```python
from build123d import *

# Parameters (mm, degrees)
SKETCH3_W            = 100
SKETCH3_H            = 120
BOSS_EXTRUDE3_DEPTH  = 4
M4_CLEARANCE_HOLE1_D = 4.5
SKETCH5_R            = 11.8
CUT_EXTRUDE3_DEPTH   = 79.204859184
FILLET1_R            = 15
SKETCH23_W           = 9
SKETCH23_H           = 10
BOSS_EXTRUDE5_DEPTH  = 10
SKETCH26_W           = 40
SKETCH26_H           = 2
BOSS_EXTRUDE6_DEPTH  = 3
SKETCH27_R           = 2.3
CUT_EXTRUDE4_DEPTH   = 6.6
CUT_EXTRUDE5_START   = -6.6
SKETCH28_R           = 2.3
CUT_EXTRUDE5_DEPTH   = 6.6
FILLET2_R            = 2
FILLET3_R            = 2
FILLET4_R            = 2
FILLET5_R            = 2
FILLET6_R            = 2
FILLET7_R            = 2


with BuildPart() as part:
    # Sketch3 → Boss-Extrude3 (new body)
    with BuildSketch(Plane(origin=(0, 0, 0), x_dir=(1, 0, 0), z_dir=(0, 1, 0))):
        Rectangle(SKETCH3_W, SKETCH3_H)
    extrude(amount=BOSS_EXTRUDE3_DEPTH)

    # M4 Clearance Hole1 (through all)
    with Locations(Plane(origin=(0, 4, 0), x_dir=(1, 0, 0), z_dir=(0, 1, 0))):
        with Locations((-8.35, -18.35), (-39.35, -18.35), (-39.35, -49.35), (-8.35, -49.35), (8.35, -18.35), (39.35, -18.35), (39.35, -49.35), (8.35, -49.35)):
            Hole(M4_CLEARANCE_HOLE1_D / 2)

    # Sketch5 → Cut-Extrude3 (cut, through all)
    with BuildSketch(Plane(origin=(0, 4, 0), x_dir=(1, 0, 0), z_dir=(0, 1, 0))):
        with Locations(Location((-23.85, -33.85, 0), (0, 0, 270))):
            Circle(SKETCH5_R)
        with Locations(Location((23.85, -33.85, 0), (0, 0, 270))):
            Circle(SKETCH5_R)
    extrude(amount=-CUT_EXTRUDE3_DEPTH, mode=Mode.SUBTRACT)

    # Fillet1
    fillet1_edges = [part.edges().sort_by_distance(p)[0] for p in [
        (50, 2, 60),
        (-50, 2, 60),
        (-50, 2, -60),
        (50, 2, -60),
    ]]
    fillet(fillet1_edges, radius=FILLET1_R)

    # Sketch23 → Boss-Extrude5 (add)
    with BuildSketch(Plane.XZ):
        with Locations((-42.5, -40)):
            Rectangle(SKETCH23_W, SKETCH23_H)
        with Locations((42.5, -40)):
            Rectangle(SKETCH23_W, SKETCH23_H)
    extrude(amount=BOSS_EXTRUDE5_DEPTH)

    # Sketch26 → Boss-Extrude6 (add)
    with BuildSketch(Plane.XZ):
        with Locations((0, 58)):
            Rectangle(SKETCH26_W, SKETCH26_H)
    extrude(amount=BOSS_EXTRUDE6_DEPTH)

    # Sketch27 → Cut-Extrude4 (cut)
    with BuildSketch(Plane.ZY.offset(47)):
        with Locations((-40, -5)):
            Circle(SKETCH27_R)
    extrude(amount=-CUT_EXTRUDE4_DEPTH, mode=Mode.SUBTRACT)

    # Sketch28 → Cut-Extrude5 (cut)
    with BuildSketch(Plane(origin=(47, 0, 0), x_dir=(0, 0, -1), z_dir=(1, 0, 0)).offset(CUT_EXTRUDE5_START)):
        with Locations(Location((40, -5, 0), (0, 0, 180))):
            Circle(SKETCH28_R)
    extrude(amount=CUT_EXTRUDE5_DEPTH, mode=Mode.SUBTRACT)

    # Fillet2
    fillet2_edges = [part.edges().sort_by_distance(p)[0] for p in [
        (38, 0, -40),
    ]]
    fillet(fillet2_edges, radius=FILLET2_R)

    # Fillet3
    fillet3_edges = [part.edges().sort_by_distance(p)[0] for p in [
        (-38, 0, -40),
    ]]
    fillet(fillet3_edges, radius=FILLET3_R)

    # Fillet4
    fillet4_edges = [part.edges().sort_by_distance(p)[0] for p in [
        (41.5, 0, -35),
    ]]
    fillet(fillet4_edges, radius=FILLET4_R)

    # Fillet5
    fillet5_edges = [part.edges().sort_by_distance(p)[0] for p in [
        (-41.5, 0, -35),
    ]]
    fillet(fillet5_edges, radius=FILLET5_R)

    # Fillet6
    fillet6_edges = [part.edges().sort_by_distance(p)[0] for p in [
        (41.5, 0, -45),
    ]]
    fillet(fillet6_edges, radius=FILLET6_R)

    # Fillet7
    fillet7_edges = [part.edges().sort_by_distance(p)[0] for p in [
        (-41.5, 0, -45),
    ]]
    fillet(fillet7_edges, radius=FILLET7_R)


solid = part.part
```
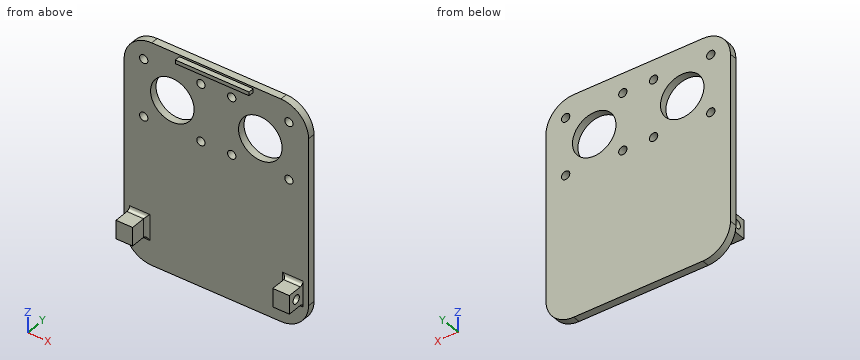
Verification items for the finished model (mm, model axes). Round coordinates to 2 decimals unless told otherwise and drop trailing zeros. Loops run counter-clockwise (first coordinate to the right, second up) from the corner with the lowest first, then second, coordinate; pieces in that order, holes last. Notation, with made-up numbers: (12, 33) -> (34, 33) arc R28 cw to (34, 51) -> close; hole circle Ø5 at (38, 69.5). An arc over 180 degrees is marked (long way). Answer as a JSON object with one key per item and string values.
Q1. Scan lines: line 1 (Z direction, x = -8.35, y = 1.1); line 2 (X direction, y = 1.05, z = 18.35); line 3 (Y direction, x = -42.5, z = -40). Record each from-to range of solid material in increasing order. Write a range as from..to.
Data:
{"line 1": "z = -60..16.1, 20.6..47.1, 51.6..60", "line 2": "x = -50..-41.6, -37.1..-10.6, -6.1..6.1, 10.6..37.1, 41.6..50", "line 3": "y = -10..-7.3, -2.7..4"}
Q2. Section check D-D (y = 2). State how many separate pieces and enclosed holes the cut face has, then the cut area to 3 significant figures.
Data:
{"separate pieces": "1", "enclosed holes": "10", "area": "10,800 mm2"}
Q3. Go/stop test with flat-tipped pins: P1, Ø2.5, axis at x = -7.5, y = -1.5, coming from the +Z side; P2, Ø3, axis at y = -5, z = -40, coming from the -X side; P3, Ø2.5, axis at x = -41.5, y = -7.5, coming from the -Z side. Record where each tip stops, or that it passes through.
Data:
{"P1": "stops at z = 59", "P2": "stops at x = -40.4", "P3": "stops at z = -45"}
Q4. Section check A-A (z = 33.85). Record the boundary of the cut face in (x, y), then the cut area to 3 significant figures.
Data:
{"outline": "(-50, 0) -> (-35.65, 0) -> (-35.65, 4) -> (-50, 4) -> close; (-12.05, 0) -> (12.05, 0) -> (12.05, 4) -> (-12.05, 4) -> close; (35.65, 0) -> (50, 0) -> (50, 4) -> (35.65, 4) -> close", "area": "211 mm2"}
Q5. Section check B-B (x = 8.35). Record the boundary of the cut face in (y, z).
Data:
{"outline": "(-3, 57) -> (0, 57) -> (0, 51.6) -> (4, 51.6) -> (4, 60) -> (0, 60) -> (0, 59) -> (-3, 59) -> close; (0, -60) -> (4, -60) -> (4, 16.1) -> (0, 16.1) -> close; (0, 20.6) -> (4, 20.6) -> (4, 47.1) -> (0, 47.1) -> close"}
Q6. Section check C-C (y = -5). Record the boundary of the cut face in (x, z).
Data:
{"outline": "(-47, -45) -> (-38, -45) -> (-38, -35) -> (-47, -35) -> (-47, -37.7) -> (-40.4, -37.7) -> (-40.4, -42.3) -> (-47, -42.3) -> close; (38, -45) -> (47, -45) -> (47, -42.3) -> (40.4, -42.3) -> (40.4, -37.7) -> (47, -37.7) -> (47, -35) -> (38, -35) -> close"}
